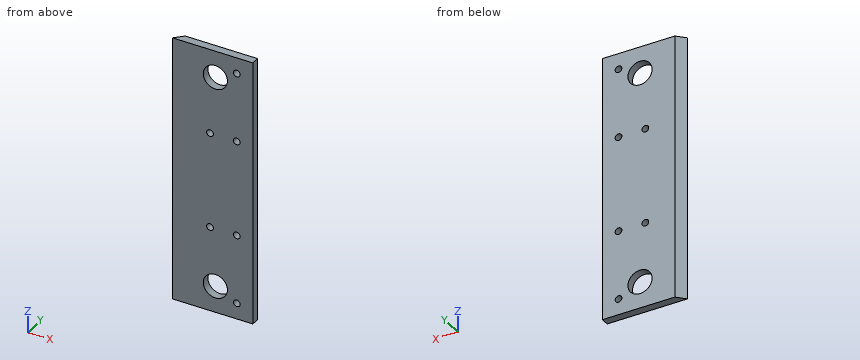
Autodesk Inventor part; units mm, degrees
ref_plane "YZ Plane" through (0, 0, 0) normal (1, 0, 0) x (0, 1, 0)
ref_plane "XZ Plane" through (0, 0, 0) normal (0, 1, 0) x (-1, 0, 0)
ref_plane "XY Plane" through (0, 0, 0) normal (0, 0, 1) x (1, 0, 0)
sketch "Sketch1" plane through (0, 0, 0) normal (0, 1, 0) x (-1, 0, 0)
  line L0 (0, 100) -> (-30, 100)
  line L1 (-30, 100) -> (-30, 0)
  line L2 (-30, 0) -> (0, 0)
  line L3 (0, 0) -> (0, 100)
  circle A0 centre (-24, 94) radius 1.25
  circle A1 centre (-24, 68) radius 1.25
  circle A2 centre (-14, 68) radius 1.25
  line L4 (-30, 50) -> (0, 50) construction
  circle A3 centre (-24, 6) radius 1.25
  circle A4 centre (-24, 32) radius 1.25
  circle A5 centre (-14, 32) radius 1.25
  circle A6 centre (-16, 90) radius 4.5
  circle A7 centre (-16, 10) radius 4.5
  dimension "d0" = 30
  dimension "d1" = 100
  dimension "d7" = 2.5
  dimension "d8" = 6
  dimension "d9" = 6
  dimension "d10" = 2.5
  dimension "d12" = 2.5
  dimension "d13" = 10
  dimension "d16" = 32
  dimension "d23" = 9
  dimension "d24" = 10
  dimension "d25" = 14
extrude "Extrusion1" add sketch "Sketch1" along normal blind 3 contours L3 L2 L1 L0 | A0 | A1 | A2 | A3 | A4 | A5 | A6 | A7
sketch "Sketch2" plane through (0, 0, 100) normal (0, 0, 1) x (1, 0, 0)
  line L0 (0, 0) -> (0, 3)
  line L1 (0, 0) -> (3, 3)
  line L2 (0, 3) -> (30, 3)
  line L3 (0, 3) -> (0, 0)
  dimension "d4" = 3
extrude "Extrusion2" cut sketch "Sketch2" against normal through all
extrude "Extrusion3" cut sketch "Sketch1" along normal through all contours A0 | A1 | A2 | A3 | A4 | A5
sketch "Sketch3" plane through (0, 3, 0) normal (0, 1, 0) x (1, 0, 0)
  circle A0 centre (16, -10) radius 4.5
  line L0 (3, 0) -> (3, -100)
  line L1 (30, 0) -> (3, 0)
  line L2 (3, -50) -> (16, -50) construction
  circle A1 centre (16, -90) radius 4.5
  line L3 (30, -100) -> (30, 0)
  point P0 (0, 0)
  dimension "d18" = 10
  dimension "d19" = 9
  dimension "d22" = 14
extrude "Extrusion4" cut sketch "Sketch3" against normal through all
properties part number "Ostrze"
Read the model definition and answer for the solid it produces. Units are mm, in the model's axes. Coordinates: 2 decimals unless noted, no trailing zeros. Order: outer loops, then holes, each group sorted by start corner. A loop starts at its lowest first (then second) coordinate and runs counter-clockwise, first axis right, second up. Notation, with made-up numbers: M -38.75,13 L -12.75,13 A33 ccw -12.75,46 Z; hole C 59.25,42 d10. An arc over 180 degrees is marked long. Put each result on its own line as item: value. Start each with the question number.
Item 1: Section B-B, the plane z = 68 is taken. Determine the outline of the cut face in (x, y), plus the area to 3 significant figures.
Item 2: Section C-C, the plane x = 24 is taken. Determine the outline of the cut face in (y, z), plus the area to 3 significant figures.
Item 3: Given pin 1 Ø2 at (x, z) = (24, 94) entering from +Y, flat-ended and moving along its own axis, determine where the tip first touches the part or whether it passes through.
Item 4: Consider probe 1 along Z at (x, y) = (16, 1.4); probe 2 along Z at (x, y) = (24, 0.9); probe 3 along X at (y, z) = (2.4, 6). Determine where each line is inside the solid, lowest interval first. Write a range as [from, to].
Item 5: Section A-A, the plane y = 1.5 is taken. Count the separate pieces of the cut face and the enclosed holes in it, plus the area to 3 significant figures.
Item 6: Section D-D, the plane x = 16.75 is taken. Determine the outline of the cut face in (y, z), plus the area to 3 significant figures.
Computed:
1. outline: M 0,0 L 12.75,0 L 12.75,3 L 3,3 Z; M 15.25,0 L 22.75,0 L 22.75,3 L 15.25,3 Z; M 25.25,0 L 30,0 L 30,3 L 25.25,3 Z
1. area: 70.5 mm2
2. outline: M 0,0 L 3,0 L 3,4.75 L 0,4.75 Z; M 0,7.25 L 3,7.25 L 3,30.75 L 0,30.75 Z; M 0,33.25 L 3,33.25 L 3,66.75 L 0,66.75 Z; M 0,69.25 L 3,69.25 L 3,92.75 L 0,92.75 Z; M 0,95.25 L 3,95.25 L 3,100 L 0,100 Z
2. area: 270 mm2
3. pin 1: passes through
4. probe 1: z = [0, 5.5], [14.5, 85.5], [94.5, 100]
4. probe 2: z = [0, 4.75], [7.25, 30.75], [33.25, 66.75], [69.25, 92.75], [95.25, 100]
4. probe 3: x = [2.4, 13.94], [18.06, 22.75], [25.25, 30]
5. separate pieces: 1
5. enclosed holes: 8
5. area: 2,690 mm2
6. outline: M 0,0 L 3,0 L 3,5.56 L 0,5.56 Z; M 0,14.44 L 3,14.44 L 3,85.56 L 0,85.56 Z; M 0,94.44 L 3,94.44 L 3,100 L 0,100 Z
6. area: 247 mm2
